For this review, use the dimensioned drawing (mm, ordinates from the lowest corner) and the shaded views. A direction names the side the tool comes from. Round coordinates to 2 decimals unless told otherwise and drop trailing zeros. Order: outer loops, then holes, each group sorted by start corner. A loop starts at its lowest first (then second) coordinate and runs counter-clockwise, first axis right, second up. Notation, with made-up numbers: (61.5, 8.25) -> (118.5, 8.25) arc R14 cw to (118.5, 22.25) -> close; hole circle Ø5 at (45.5, -23.5). An arc over 180 degrees is marked (long way). Use a Markdown table: item, result. Add a question column.
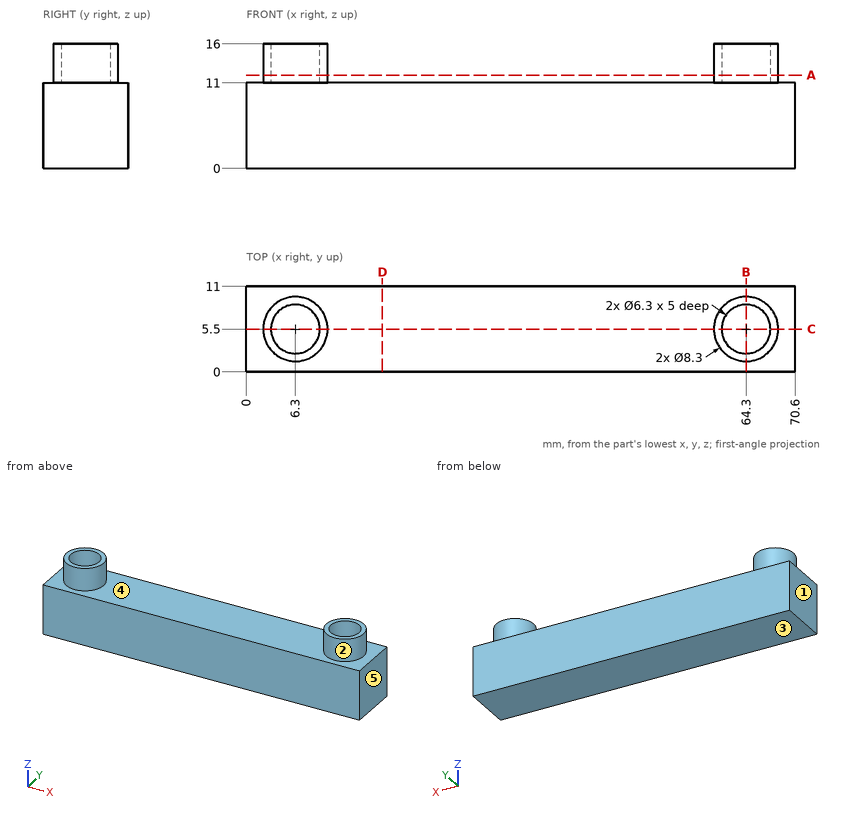
Q1. Add section C-C (y = 5.5). Write out the cut boundary in (x, z).
Q2. Add section B-B (x = 64.3). Write out the cut boundary in (y, z).
Q3. Add section D-D (x = 17.5). Write out the cut boundary in (y, z).
Q4. Add section A-A (z = 12). Write out the cut boundary in (x, y), then the cut area to 3 significant figures.
Q5. Machinability: for the marked faces 1 and 2, which of the approach directions +Z, -Z, +X, -X, +Y, -Y give a long, thin tool a straight path to every point of the face, cutting with its end or side? Answer none if there is none.
Q6. Mouldability with a two-part tool opening along X and no side actions: class the marked faces 3, 4 and 5 as pulls with the +X half, pulls with the -X half, needs draft (parallel to the pull), parting line crosses it, or undercut.
Q7. Insertion check: pin 1 (5 mm diameter, centred on x = 64.3, y = 5.5, fed in from +Z). The pin has a flat end and moves straight along its axis. Give the tip position at first contact, or say it passes through.
Q8. Wall thickness on line 1 (X direction, y = 5.75, z = 12.75); line 2 (Y direction, x = 64.3, z = 13.4); line 3 (X direction, y = 7.75, z = 11.25): over which ranges is each line inside the solid? List them lowest first. Write a range as [from, to].
Report:
| question | item | result |
|---|---|---|
| 1 | outline | (0, 0) -> (70.6, 0) -> (70.6, 11) -> (68.45, 11) -> (68.45, 16) -> (67.45, 16) -> (67.45, 11) -> (61.15, 11) -> (61.15, 16) -> (60.15, 16) -> (60.15, 11) -> (10.45, 11) -> (10.45, 16) -> (9.45, 16) -> (9.45, 11) -> (3.15, 11) -> (3.15, 16) -> (2.15, 16) -> (2.15, 11) -> (0, 11) -> close |
| 2 | outline | (0, 0) -> (11, 0) -> (11, 11) -> (9.65, 11) -> (9.65, 16) -> (8.65, 16) -> (8.65, 11) -> (2.35, 11) -> (2.35, 16) -> (1.35, 16) -> (1.35, 11) -> (0, 11) -> close |
| 3 | outline | (0, 0) -> (11, 0) -> (11, 11) -> (0, 11) -> close |
| 4 | outline | circle Ø8.3 at (6.3, 5.5); circle Ø8.3 at (64.3, 5.5); hole circle Ø6.3 at (6.3, 5.5); hole circle Ø6.3 at (64.3, 5.5) |
| 4 | area | 45.9 mm² |
| 5 | face 1 | +Z, -Z, -X, +Y, -Y |
| 5 | face 2 | +Z |
| 6 | face 3 | needs draft |
| 6 | face 4 | undercut |
| 6 | face 5 | pulls with the +X half |
| 7 | pin 1 | stops at z = 11 |
| 8 | line 1 | x = [2.16, 3.16], [9.44, 10.44], [60.16, 61.16], [67.44, 68.44] |
| 8 | line 2 | y = [1.35, 2.35], [8.65, 9.65] |
| 8 | line 3 | x = [2.81, 4.1], [8.5, 9.79], [60.81, 62.1], [66.5, 67.79] |
